Input: dimensioned drawing with shaded views. Units: mm. Origin: part minimum x, y, z. Round coordinates to 2 decimals unless told otherwise and drop trailing zeros. Write each loop counter-clockwise with the first axis right and the second up, starting at its lowest first coordinate (ties: lowest second). Pieces come first, ordered by that corner, then holes. Notation, with made-up numbers: (16, 86) - (26, 86) arc R24 ccw to (26, 122) - close; hole circle Ø6 at (52.25, 39). An arc over 180 degrees is marked (long way). Write item = value, one per line. Start each with the question number.
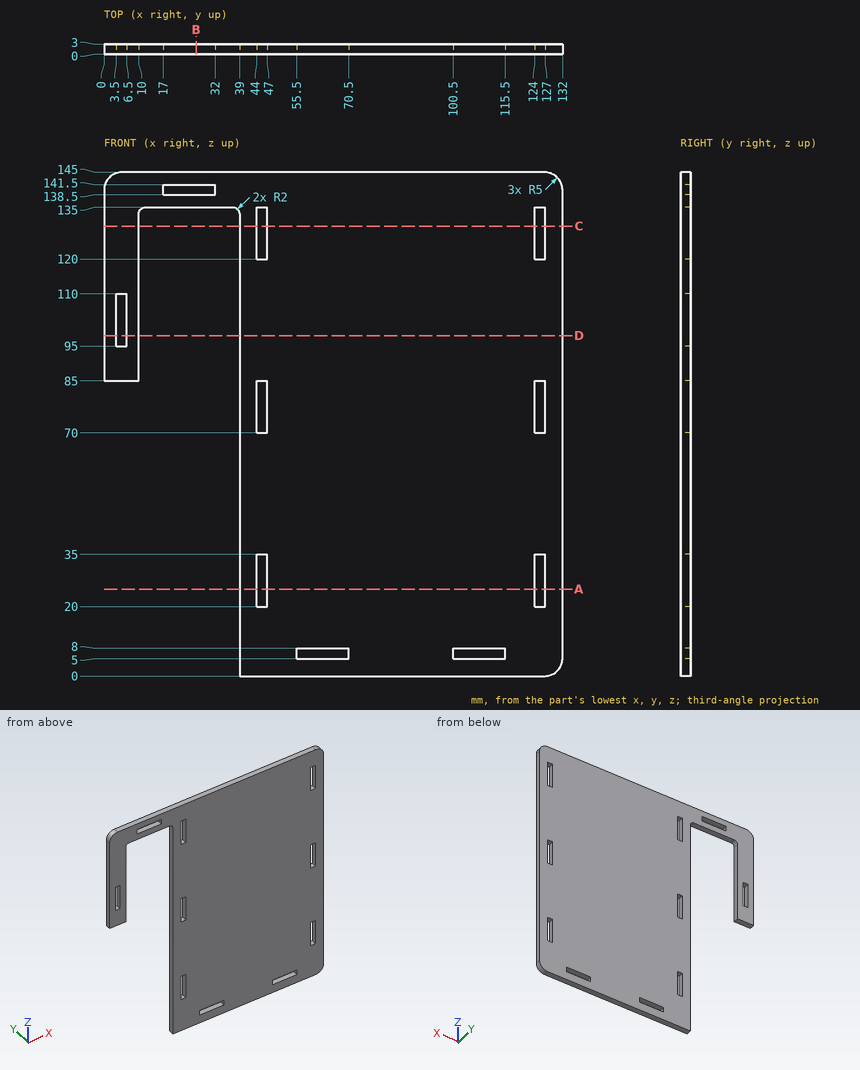
(1) Section C-C (z = 129.5). Return the cut outline in (x, y).
(2) Section D-D (z = 98). Return the cut outline in (x, y).
(3) Ray query, L1, parallel to X at y = 1.65, z = 32.5; L2, parallel to X at y = 1.8, z = 101; L3, parallel to Z at x = 113, y = 0.7. Return the intervals inside material, ascending. Write a range as from..to.
(4) Contact query for flat-ended pins moving along their axis: P1, Ø0.9, axis at x = 7, y = 1.5, coming from the -Z side; P2, Ø1, axis at y = 2.5, z = 38, coming from the -X side. Output: stop coordinate, or through.
(5) Section A-A (z = 25). Return the cut outline in (x, y).
(6) Section B-B (x = 26.5). Return the cut outline in (y, z), plus the area to 3 significant figures.
Solution:
q1.outline = (0, 0) - (10, 0) - (10, 3) - (0, 3) - close; (39, 0) - (44, 0) - (44, 3) - (39, 3) - close; (47, 0) - (124, 0) - (124, 3) - (47, 3) - close; (127, 0) - (132, 0) - (132, 3) - (127, 3) - close
q2.outline = (0, 0) - (3.5, 0) - (3.5, 3) - (0, 3) - close; (6.5, 0) - (10, 0) - (10, 3) - (6.5, 3) - close; (39, 0) - (132, 0) - (132, 3) - (39, 3) - close
q3.L1 = 39..44, 47..124, 127..132
q3.L2 = 0..3.5, 6.5..10, 39..132
q3.L3 = 0..5, 8..145
q4.P1 = 85
q4.P2 = 39
q5.outline = (39, 0) - (44, 0) - (44, 3) - (39, 3) - close; (47, 0) - (124, 0) - (124, 3) - (47, 3) - close; (127, 0) - (132, 0) - (132, 3) - (127, 3) - close
q6.outline = (0, 135) - (3, 135) - (3, 138.5) - (0, 138.5) - close; (0, 141.5) - (3, 141.5) - (3, 145) - (0, 145) - close
q6.area = 21.0 mm^2
